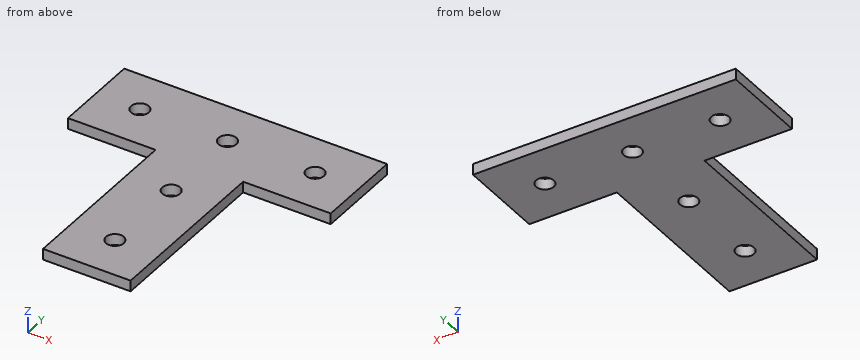
Autodesk Inventor part; units mm, degrees
ref_plane "YZ Plane" through (0, 0, 0) normal (1, 0, 0) x (0, 1, 0)
ref_plane "XZ Plane" through (0, 0, 0) normal (0, 1, 0) x (-1, 0, 0)
ref_plane "XY Plane" through (0, 0, 0) normal (0, 0, 1) x (1, 0, 0)
sketch "Sketch1" plane through (0, 0, 0) normal (0, 0, 1) x (1, 0, 0)
  line L0 (76.2, 0) -> (76.2, 25.4)
  line L1 (76.2, 25.4) -> (0, 25.4)
  line L2 (0, 25.4) -> (0, 0)
  line L3 (0, 0) -> (25.4, 0) construction
  line L4 (25.4, 0) -> (25.4, -50.8)
  line L5 (25.4, -50.8) -> (50.8, -50.8)
  line L6 (50.8, -50.8) -> (50.8, 0)
  line L7 (0, 0) -> (25.4, 0)
  line L8 (50.8, 0) -> (76.2, 0)
  line L9 (0, 12.7) -> (12.7, 12.7) construction
  line L10 (12.7, 12.7) -> (38.1, 12.7) construction
  line L11 (38.1, 12.7) -> (63.5, 12.7) construction
  line L12 (38.1, 12.7) -> (38.1, -12.7) construction
  line L13 (38.1, -12.7) -> (38.1, -38.1) construction
  circle A0 centre (12.7, 12.7) radius 2.5781
  circle A1 centre (38.1, 12.7) radius 2.5781
  circle A2 centre (63.5, 12.7) radius 2.5781
  circle A3 centre (38.1, -12.7) radius 2.5781
  circle A4 centre (38.1, -38.1) radius 2.5781
  dimension "d0" = 76.2
  dimension "d1" = 25.4
  dimension "d2" = 25.4
  dimension "d3" = 50.8
  dimension "d4" = 25.4
  dimension "d5" = 25.4
  dimension "d6" = 25.4
  dimension "d7" = 5.1562
extrude "Extrusion1" add sketch "Sketch1" along normal blind 3.175
properties part number "T-Gusset"
Here's how the part is built. I have some questions about the finished solid (model axes, mm). Round coordinates to 2 decimals unless told otherwise and drop trailing zeros. Loops run counter-clockwise (first coordinate to the right, second up) from the corner with the lowest first, then second, coordinate; pieces in that order, holes last. Notation, with made-up numbers: (70.25, 55) -> (112.25, 55) arc R21 cw to (112.25, 67) -> close; hole circle Ø8 at (43.5, 46). An arc over 180 degrees is marked (long way). Answer as CSV lines item,"result".
1. If I drill on L1, parallel to Y at x = 38.1, z = 1.65; L2, parallel to Y at x = 40, z = 2.9; L3, parallel to Y at x = 12.7, z = 2.3, over which ranges is the centre line in solid material (lowest first)?
Final values:
L1,"y = -50.8 to -40.68, -35.52 to -15.28, -10.12 to 10.12, 15.28 to 25.4"
L2,"y = -50.8 to -39.84, -36.36 to -14.44, -10.96 to 10.96, 14.44 to 25.4"
L3,"y = 0 to 10.12, 15.28 to 25.4"
2. For pin 1 (1.6 mm diameter, centred on y = -31, z = 1, fed in from +X); pin 2 (1.6 mm diameter, centred on x = 69, z = 1.5, fed in from -Y), each with a flat end and sliding along its axis, tell me the tip position at first contact or that it passes through.
Final values:
pin 1,"stops at x = 50.8"
pin 2,"stops at y = 0"
3. If we section it at D-D on x = 63.5: Please give me the cut outline in (y, z) (3 decimals), plus the area to 3 significant figures.
Final values:
outline,"(0, 0) -> (10.122, 0) -> (10.122, 3.175) -> (0, 3.175) -> close; (15.278, 0) -> (25.4, 0) -> (25.4, 3.175) -> (15.278, 3.175) -> close"
area,"64.3 mm^2"
4. If we section it at C-C on z = 1.05: Please give me the cut outline in (x, y), plus the area to 3 significant figures.
Final values:
outline,"(0, 0) -> (25.4, 0) -> (25.4, -50.8) -> (50.8, -50.8) -> (50.8, 0) -> (76.2, 0) -> (76.2, 25.4) -> (0, 25.4) -> close; hole circle Ø5.16 at (12.7, 12.7); hole circle Ø5.16 at (38.1, -38.1); hole circle Ø5.16 at (38.1, -12.7); hole circle Ø5.16 at (38.1, 12.7); hole circle Ø5.16 at (63.5, 12.7)"
area,"3,120 mm^2"
5. If we section it at A-A on y = -12.7: Please give me the cut outline in (x, z) (3 decimals).
Final values:
outline,"(25.4, 0) -> (35.522, 0) -> (35.522, 3.175) -> (25.4, 3.175) -> close; (40.678, 0) -> (50.8, 0) -> (50.8, 3.175) -> (40.678, 3.175) -> close"
6. If we section it at B-B on x = 38.1: Please give me the cut outline in (y, z) (3 decimals).
Final values:
outline,"(-50.8, 0) -> (-40.678, 0) -> (-40.678, 3.175) -> (-50.8, 3.175) -> close; (-35.522, 0) -> (-15.278, 0) -> (-15.278, 3.175) -> (-35.522, 3.175) -> close; (-10.122, 0) -> (10.122, 0) -> (10.122, 3.175) -> (-10.122, 3.175) -> close; (15.278, 0) -> (25.4, 0) -> (25.4, 3.175) -> (15.278, 3.175) -> close"
